Build history of the part. All positions in model axes, mm. A direction names the side the tool comes from. Give positions to 0.01 mm unless a question says otherwise; leave off trailing zeros. Order: outer loops, then holes, each group sorted by start corner. A loop starts at its lowest first (then second) coordinate and runs counter-clockwise, first axis right, second up. Notation, with made-up numbers: M 72.25,-19.5 L 101.25,-19.5 A24 cw 101.25,4.5 Z; hole C -20.75,-20.5 d5. An arc over 180 degrees is marked long. One line per item, written item: value.
from build123d import *

# Parameters (mm, degrees)
BOSS_EXTRUDE1_DEPTH = 288.29
CUT_EXTRUDE2_REACH  = 301.942
SKETCH4_W           = 7.62
SKETCH4_H           = 23.8125
LPATTERN1_COUNT     = 3
LPATTERN1_PITCH     = 76.2
SKETCH5_R           = 1.3890625
CUT_EXTRUDE3_DEPTH  = 14.2875
LPATTERN2_COUNT     = 3
LPATTERN2_PITCH     = 76.2


with BuildPart() as part:
    # Sketch1 → Boss-Extrude1 (new body)
    with BuildSketch(Plane.XY):
        Polygon((57.15, 0), (57.15, 31.75), (6.35, 31.75), (6.35, 0), (0, 0), (0, 31.75), (-10, 31.75), (-10, 38.1), (0, 38.1), (63.5, 38.1), (73.5, 38.1), (73.5, 31.75), (63.5, 31.75), (63.5, 9.525), (63.5, 0), align=None)
    extrude(amount=BOSS_EXTRUDE1_DEPTH)

    # Cut-Extrude2: up to this face of the body (flat: up to its plane)
    cut_extrude2_end = Plane(part.part.faces().sort_by_distance((0, 15.875, 144.145))[0])
    # Sketch4 → Cut-Extrude2 (cut, up to the picked face)
    with BuildSketch(Plane(origin=(63.5, 0, 0), x_dir=(0, 0, -1), z_dir=(1, 0, 0)), mode=Mode.PRIVATE) as cut_extrude2_sk1:
        with Locations((-220.345, 11.90625)):
            Rectangle(SKETCH4_W, SKETCH4_H)
    cut_extrude2_tool1 = split(extrude(cut_extrude2_sk1.sketch, amount=-CUT_EXTRUDE2_REACH, mode=Mode.PRIVATE), bisect_by=cut_extrude2_end, keep=Keep.BOTH, mode=Mode.PRIVATE)
    cut_extrude2 = cut_extrude2_tool1.solids().sort_by(Axis((63.5, 11.90625, 220.345), (-1, 0, 0)))[0]
    add(cut_extrude2, mode=Mode.SUBTRACT)

    # LPattern1: Cut-Extrude2 ×3
    with Locations(*[(0, 0, -i * LPATTERN1_PITCH) for i in range(1, LPATTERN1_COUNT)]):
        add(cut_extrude2, mode=Mode.SUBTRACT)

    # Sketch5 → Cut-Extrude3 (cut)
    with BuildSketch(Plane(origin=(0, 38.1, 0), x_dir=(1, 0, 0), z_dir=(0, 1, 0))):
        with Locations(Location((60.325, -220.345, 0), (0, 0, 270))):
            Circle(SKETCH5_R)
        with Locations(Location((3.175, -220.345, 0), (0, 0, 270))):
            Circle(SKETCH5_R)
    cut_extrude3 = extrude(amount=-CUT_EXTRUDE3_DEPTH, mode=Mode.SUBTRACT)

    # LPattern2: Cut-Extrude3 ×3
    with Locations(*[(0, 0, -i * LPATTERN2_PITCH) for i in range(1, LPATTERN2_COUNT)]):
        add(cut_extrude3, mode=Mode.SUBTRACT)


solid = part.part
1) Saw through at D-D, the plane x = 51. Write the cut outline in (y, z).
Check values:
outline: M 31.75,0 L 38.1,0 L 38.1,288.29 L 31.75,288.29 Z
2) Mould opens along Z. For faces 1 (the face through (60, 12, 216.535)), 2 (the face through (60, 0, 32)), 3 (the face through (60, 12, 71.755)) say: released by +Z, released by -Z, zero draft, split by the parting line, or undercut.
Check values:
face 1: undercut
face 2: zero draft
face 3: undercut
3) Tool access for faces 4 (the face through (57.15, 26, 142)), 5 (the face through (32, 38.1, 142)), 6 (the face through (63.5, 26, 142)), 7 (the face through (-10, 35, 142)), 8 (the face through (60, 12, 147.955)): list every direction of +Z, -Z, +X, -X, +Y, -Y with a clear straight run to the whole face (end or side of a thin tool).
Check values:
face 4: +Z, -Z, -Y
face 5: +Z, -Z, +X, -X, +Y
face 6: +Z, -Z, +X, -Y
face 7: +Z, -Z, -X, +Y, -Y
face 8: +X, -X, -Y
4) Saw through at B-B, the plane y = 27.5. Write the cut outline in (x, z) (3 decimals), then the cut area to 3 significant figures.
Check values:
outline: M 0,0 L 6.35,0 L 6.35,288.29 L 0,288.29 Z; M 57.15,0 L 63.5,0 L 63.5,288.29 L 57.15,288.29 Z; hole C 3.175,67.945 d2.778; hole C 3.175,144.145 d2.778; hole C 3.175,220.345 d2.778; hole C 60.325,67.945 d2.778; hole C 60.325,144.145 d2.778; hole C 60.325,220.345 d2.778
area: 3,620 mm^2
5) Pin check, flat tips, straight feed: pin 1 (1.9 mm diameter, centred on x = 2.5, z = 67, fed in from -Y); pin 2 (1 mm diameter, centred on x = 20, z = 257.5, fed in from -Y); pin 3 (1.5 mm diameter, centred on y = 4.5, z = 156.5, fed in from +X); pin 4 (3 mm diameter, centred on x = 55.5, y = 16.5, fed in from -Z). Stop position of each tip, or through.
Check values:
pin 1: y = 23.81
pin 2: y = 31.75
pin 3: x = 63.5
pin 4: through
6) Saw through at C-C, the plane z = 185. Write the cut outline in (x, y).
Check values:
outline: M -10,31.75 L 0,31.75 L 0,0 L 6.35,0 L 6.35,31.75 L 57.15,31.75 L 57.15,0 L 63.5,0 L 63.5,31.75 L 73.5,31.75 L 73.5,38.1 L -10,38.1 Z
7) Drill centre lines: probe 1 along Z at (x, y) = (1.5, 19) (3 decimals); probe 2 along X at (y, z) = (12, 149); probe 3 along Z at (x, y) = (59.5, 24). Where is each one in solid material? Low to high. Write a range as from..to.
Check values:
probe 1: 0..64.135, 71.755..140.335, 147.955..216.535, 224.155..288.29
probe 2: 0..6.35, 57.15..63.5
probe 3: 0..66.83, 69.06..143.03, 145.26..219.23, 221.46..288.29
8) Saw through at A-A, the plane y = 3. Give the number of separate pieces and of enclosed holes in the cut face, then the cut area to 3 significant figures.
Check values:
separate pieces: 8
enclosed holes: 0
area: 3,370 mm^2
